Autodesk Fusion 360 part; units mm, degrees
sketch "Esquisse1" plane through (0, 0, 0) normal (1, 0, 0) x (0, 1, 0)
  line L0 (13.5, 3) -> (13.5, 0)
  line L1 (13.5, 0) -> (14.5, 0)
  line L2 (14.5, 0) -> (14.5, 5)
  line L3 (14.5, 5) -> (9, 5)
  line L4 (9, 15) -> (8.5, 15)
  line L5 (8.5, 15) -> (8.5, 47)
  line L6 (8.5, 47) -> (0, 47)
  line L7 (0, 47) -> (0, 3)
  line L8 (0, 3) -> (13.5, 3)
  line L9 (9, 15) -> (9, 5)
  dimension "d33" = 3
  dimension "d34" = 13.5
  dimension "d35" = 1
  dimension "d36" = 5
  dimension "d40" = 32
  dimension "d41" = 8.5
  dimension "d43" = 9
  dimension "d44" = 10
revolve "Révolution1" add sketch "Esquisse1" angle 360 about axis through (0, 0, 47) along (0, 0, -1)
sketch "Esquisse1 (2)" plane through (0, 0, 5) normal (0, 0, 1) x (-1, 0, 0)
sketch "Esquisse2" plane through (0, 0, 5) normal (0, 0, 1) x (1, 0, 0)
  circle A0 centre (0, 0) radius 11.75 construction
  circle A1 centre (0, -11.75) radius 1.5
  dimension "d57" = 23.5
  dimension "d58" = 3
extrude "Extrusion1" cut sketch "Esquisse2" against normal blind 4
pattern_circular "Réseau C1" count 3 over 360 about axis through (0, 0, 47) along (0, 0, -1) of "Extrusion1"
equation "d41 = ( 17 / 2 ) * 1 mm"
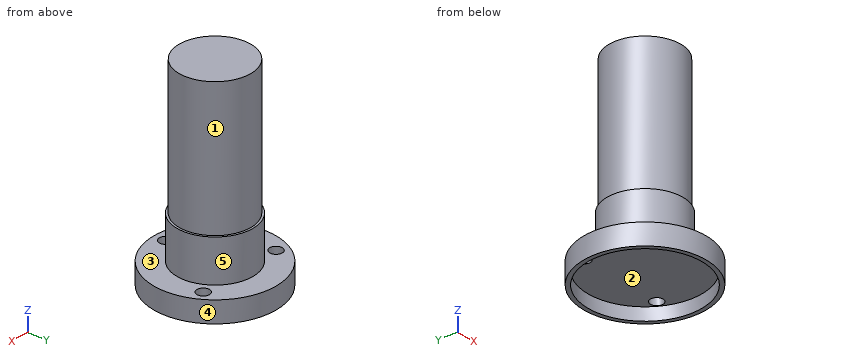
Build history of the part. All positions in model axes, mm. Face numbers are marked on the shaded views. A direction names the side the tool comes from. Round coordinates to 2 decimals unless told otherwise and drop trailing zeros. Order: outer loops, then holes, each group sorted by start corner. A loop starts at its lowest first (then second) coordinate and runs counter-clockwise, first axis right, second up. Notation, with made-up numbers: M 11,52 L 68,52 A30 cw 68,85 Z; hole C 42,57 d11. An arc over 180 degrees is marked long. Use CSV: the item, a comma, the result in double quotes. Start each with the question number.
(1) Cut at B-B on y = 5.5. List the corners of the cut face in (x, z), then the cut area to 3 significant figures.
(2) Cut at C-C on y = -11.75. List the corners of the cut face in (x, z).
(3) Cut at D-D on z = 15.5. List the corners of the cut face in (x, y), then the cut area to 3 significant figures.
(4) Flat gauge pins, fed straight in: P1, Ø1, axis at x = 11.5, y = 3, coming from the +Z side; P2, Ø3, axis at x = -5.5, z = 19, coming from the +Y side; P3, Ø12, axis at x = -1.5, z = 35, coming from the +Y side. Where does each tip first touch, or does it go through?
(5) Tool access for the marked faces 4 and 5: list every direction of +Z, -Z, +X, -X, +Y, -Y with a clear straight run to the whole face (end or side of a thin tool).
(6) Cut at A-A on x = 0. List the corners of the cut face in (y, z).
(7) Drill centre lines: probe 1 along Z at (x, y) = (-0.75, 8.5); probe 2 along Z at (x, y) = (-5.5, 2.75); probe 3 along Y at (x, z) = (6, 40.5). Where is each one in solid material? Low to high.
(8) Mould opens along Y. For the marked faces 1, 2 and 3 say: +Y half, -Y half, draft (parallel to the pull), parting line (faces both ways), or undercut.
Findings:
1,outline,"M -13.42,0 L -12.33,0 L -12.33,3 L -11.63,3 L -11.63,5 L -13.42,5 Z; M -8.72,3 L 8.72,3 L 8.72,5 L 7.12,5 L 7.12,15 L 6.48,15 L 6.48,47 L -6.48,47 L -6.48,15 L -7.12,15 L -7.12,5 L -8.72,5 Z; M 11.63,3 L 12.33,3 L 12.33,0 L 13.42,0 L 13.42,5 L 11.63,5 Z"
1,area,"606 mm^2"
2,outline,"M -8.5,0 L -6.65,0 L -6.65,3 L -1.5,3 L -1.5,5 L -8.5,5 Z; M 1.5,3 L 6.65,3 L 6.65,0 L 8.5,0 L 8.5,5 L 1.5,5 Z"
3,outline,"C 0,0 d17"
3,area,"227 mm^2"
4,P1,"stops at z = 5"
4,P2,"stops at y = 7.5"
4,P3,"stops at y = 8.5"
5,face 4,"+Z, -Z"
5,face 5,"+Z"
6,outline,"M -14.5,0 L -13.5,0 L -13.5,3 L -13.25,3 L -13.25,5 L -14.5,5 Z; M -10.25,3 L 13.5,3 L 13.5,0 L 14.5,0 L 14.5,5 L 9,5 L 9,15 L 8.5,15 L 8.5,47 L -8.5,47 L -8.5,15 L -9,15 L -9,5 L -10.25,5 Z"
7,probe 1,"z = 3 to 15"
7,probe 2,"z = 3 to 47"
7,probe 3,"y = -6.02 to 6.02"
8,face 1,"parting line"
8,face 2,"undercut"
8,face 3,"draft"
